```python
from build123d import *

# Parameters (mm, degrees)
SKETCH_1_R      = 10.5
SKETCH_1_R_2    = 6
EXTRUDE_1_DEPTH = 5
FILLET_1_R      = 1
CHAMFER_1_SIZE  = 1


with BuildPart() as part:
    # Эскиз1 → Бобышка-Вытянуть1 (new body)
    with BuildSketch(Plane(origin=(0, 0, 0), x_dir=(1, 0, 0), z_dir=(0, 1, 0))):
        Circle(SKETCH_1_R)
        Circle(SKETCH_1_R_2, mode=Mode.SUBTRACT)
    extrude(amount=EXTRUDE_1_DEPTH)

    # Скругление1
    fillet_1_edges = [part.edges().sort_by_distance(p)[0] for p in [
        (-6, 0, 0),
        (-6, 5, 0),
    ]]
    fillet(fillet_1_edges, radius=FILLET_1_R)

    # Фаска1
    chamfer_1_edges = [part.edges().sort_by_distance(p)[0] for p in [
        (-10.5, 0, 0),
        (-10.5, 5, 0),
    ]]
    chamfer(chamfer_1_edges, length=CHAMFER_1_SIZE)


solid = part.part
```
Source: CAD feature listing. Evaluate the final solid. Frame: model axes, mm. Round coordinates to 2 decimals unless told otherwise and drop trailing zeros. Write each loop counter-clockwise with the first axis right and the second up, starting at its lowest first coordinate (ties: lowest second). Pieces come first, ordered by that corner, then holes. Notation, with made-up numbers: M 38,42 L 46,42 A12 cw 46,60 Z; hole C 40,22 d11. An arc over 180 degrees is marked long. Use CSV: the item, a comma, the result in double quotes. Start each with the question number.
Q1. First-contact query: P1, Ø1.5, axis at y = 2.5, z = 2.5, coming from the -X side; P2, Ø2, axis at y = 2, z = -2, coming from the -X side; P3, Ø2, axis at x = -7.5, y = 4, coming from the +Z side. Flat tips, straight axial feed; report the tip coordinate or a pass-through.
Q2. Cut plane D-D on y = 0.5. Output: boundary loops of the cut face in (x, z), plus the area to 3 significant figures.
Q3. Cut plane C-C on y = 2.8. Output: boundary loops of the cut face in (x, z).
Q4. Pull-direction query (Z, two-part tool) for faces 1 (the face through (10, 2.5, -3.2)), 2 (the face through (-6, 2, 0)), 3 (the face through (-4, 0, 6)); classes: +Z half, -Z half, draft (parallel to the pull), parting line (faces both ways), or undercut.
Q5. Cut plane A-A on x = 0. Output: boundary loops of the cut face in (y, z).
Q6. Cut plane B-B on z = 0. Output: boundary loops of the cut face in (x, y).
Q7. Line query: line 1 (Z direction, x = 0, y = 3.05); line 2 (X direction, y = 2.25, z = -2.25). Output: solid intervals per line, ascending. Write a range as from..to.
Results found:
1,P1,"x = -10.35"
1,P2,"x = -10.45"
1,P3,"z = 8.25"
2,outline,"C 0,0 d20; hole C 0,0 d12.27"
2,area,"196 mm^2"
3,outline,"C 0,0 d21; hole C 0,0 d12"
4,face 1,"parting line"
4,face 2,"undercut"
4,face 3,"draft"
5,outline,"M 0,-9.5 L 1,-10.5 L 4,-10.5 L 5,-9.5 L 5,-7 A1 ccw 4,-6 L 1,-6 A1 ccw 0,-7 Z; M 0,7 A1 ccw 1,6 L 4,6 A1 ccw 5,7 L 5,9.5 L 4,10.5 L 1,10.5 L 0,9.5 Z"
6,outline,"M -10.5,1 L -9.5,0 L -7,0 A1 ccw -6,1 L -6,4 A1 ccw -7,5 L -9.5,5 L -10.5,4 Z; M 6,1 A1 ccw 7,0 L 9.5,0 L 10.5,1 L 10.5,4 L 9.5,5 L 7,5 A1 ccw 6,4 Z"
7,line 1,"-10.5..-6, 6..10.5"
7,line 2,"-10.26..-5.56, 5.56..10.26"
